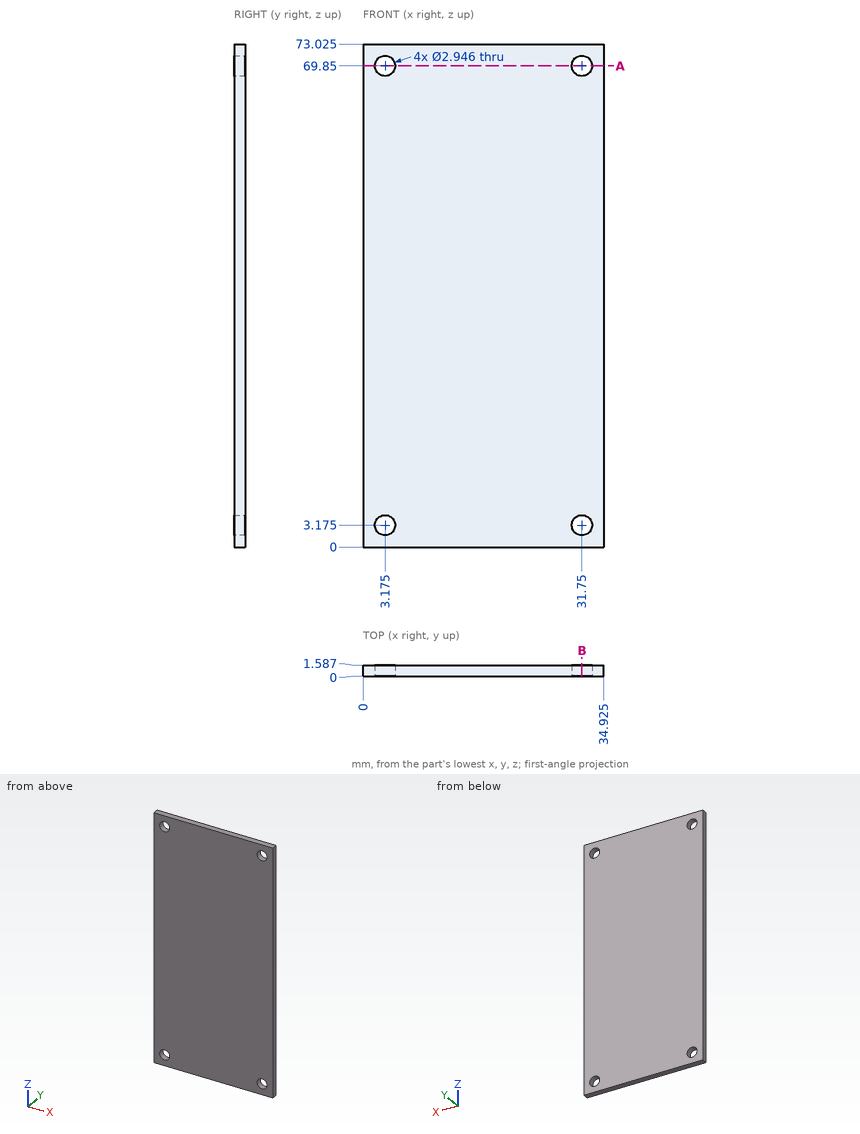
Print and shaded views of the part. All mm, measured from the part's lowest x, y and z. Coordinates: 2 decimals unless noted, no trailing zeros. Loops run counter-clockwise (first coordinate to the right, second up) from the corner with the lowest first, then second, coordinate; pieces in that order, holes last. Notation, with made-up numbers: (-28.5, 1) - (-22.5, 1) arc R18 ccw to (-22.5, 17) - close; hole circle Ø8 at (10, 88). An arc over 180 degrees is marked (long way). Write item = value, one per line. Start each with the question number.
Item 1: Saw through at B-B, the plane x = 31.75. List the corners of the cut face in (y, z) (1 decimal).
Item 2: Saw through at A-A, the plane z = 69.85. List the corners of the cut face in (x, y) (1 decimal).
Item 3: Drop flat-ended pins along their axis: pin 1 Ø1.8 at (x, z) = (3.175, 69.85) entering from +Y; pin 2 Ø3.5 at (x, z) = (31.75, 3.175) entering from -Y. Give the stop position or say it passes through.
Item 4: Wall check: probe 1 along X at (y, z) = (0.8, 69.85) (1 decimal); probe 2 along Z at (x, y) = (3, 0.9) (1 decimal); probe 3 along Z at (x, y) = (31, 1.1) (1 decimal). Give the ranges that are in metal, low to high. Write a range as [from, to].
Answers:
q1.outline = (0, 0) - (1.6, 0) - (1.6, 1.7) - (0, 1.7) - close; (0, 4.6) - (1.6, 4.6) - (1.6, 68.4) - (0, 68.4) - close; (0, 71.3) - (1.6, 71.3) - (1.6, 73) - (0, 73) - close
q2.outline = (0, 0) - (1.7, 0) - (1.7, 1.6) - (0, 1.6) - close; (4.6, 0) - (30.3, 0) - (30.3, 1.6) - (4.6, 1.6) - close; (33.2, 0) - (34.9, 0) - (34.9, 1.6) - (33.2, 1.6) - close
q3.pin_1 = through
q3.pin_2 = 0
q4.probe_1 = [0, 1.7], [4.6, 30.3], [33.2, 34.9]
q4.probe_2 = [0, 1.7], [4.6, 68.4], [71.3, 73]
q4.probe_3 = [0, 1.9], [4.4, 68.6], [71.1, 73]
